The listing builds one solid part. Answer for the finished solid, in the listing's coordinates (mm). A direction names the side the tool comes from. Give positions to 0.01 mm unless a question says otherwise; leave off trailing zeros. Loops run counter-clockwise (first coordinate to the right, second up) from the corner with the lowest first, then second, coordinate; pieces in that order, holes last. Notation, with made-up numbers: M 25,69 L 84,69 A23 cw 84,79 Z; hole C 74,24 d3. An arc over 180 degrees is marked long. One line per item, written item: value. Start each with the question number.
Q1. A cutting plane is placed at A-A, the plane x = -1.25. Determine the outline of the cut face in (y, z), and give its area (3 significant figures).
Q2. For faces 5 (the cylindrical face through (2.84, -3.63, 0.22)), 6 (the cylindrical face through (-0.518, -0.045, 1.377)), 7 (the cylindrical face through (2.39, 0.07, -5.72)), 8 (the cylindrical face through (-1.644, -1.029, 1.643)), 9 (the flat face through (-6.422, 0, 1)), determine the directions among +Z, -Z, +X, -X, +Y, -Y from which every point of the face is accessible in a straight line to the end or side of a thin tool.
Q3. Flat-ended cylindrical pins translate along their axes: pin 1 (6 mm diameter, centred on x = 0, z = -0.956, fed in from -Y); pin 2 (1.6 mm diameter, centred on x = 4.5, y = 0, fed in from -Z); pin 3 (1.3 mm diameter, centred on x = 3.5, y = -1, fed in from +Z). Find the tip coordinate at first contact, or state that the pin passes through.
Q4. A cutting plane is placed at D-D, the plane x = 5.5. Determine the outline of the cut face in (y, z).
Q5. The mould has two halves that part along Z. Classify faces 1 (the flat face through (0, 0, -4.839)), 2 (the flat face through (0, 0, 4.839)), 3 (the flat face through (4, 0, -3.197)), 4 (the cylindrical face through (-1.567, 0.493, 3.219)): +Z half, -Z half, draft (parallel to the pull), parting line (faces both ways), or undercut.
Q6. A cutting plane is placed at C-C, the plane z = -3. Determine the outline of the cut face in (x, y) (1 decimal).
Q7. Consider L1, parallel to Y at x = -5, z = -2.25; L2, parallel to Z at x = 0, y = 3.8; L3, parallel to X at y = 0.25, z = 0.25 (1 decimal). Determine where each line is inside the solid, lowest interval first.
from build123d import *

# Parameters (mm, degrees)
SKETCH1_W                = 16.13
SKETCH1_H                = 9.678
BOSS_EXTRUDE1_DEPTH      = 8.065
SKETCH2_W                = 12.845
SKETCH2_H                = 4.78
CUT_EXTRUDE1_DEPTH       = 8.0355
BOSS_EXTRUDE2_DEPTH      = 4.78
SKETCH4_W                = 2.39
SKETCH4_H                = 1.78
SKETCH5_W                = 2.39
SKETCH5_H                = 1.78
SKETCH7_W                = 1.6425
SKETCH7_H                = 3.195419505
M3_CLEARANCE_HOLE1_D     = 3.285
M3_CLEARANCE_HOLE1_DEPTH = 1.78


with BuildPart() as part:
    # Sketch1 → Boss-Extrude1 (new body)
    with BuildSketch(Plane(origin=(0, 4.0325, 0), x_dir=(-1, 0, 0), z_dir=(0, 1, 0))):
        Rectangle(SKETCH1_W, SKETCH1_H)
    extrude(amount=-BOSS_EXTRUDE1_DEPTH)

    # Sketch2 → Cut-Extrude1 (cut)
    with BuildSketch(Plane.XY.offset(4.839)):
        Rectangle(SKETCH2_W, SKETCH2_H)
    extrude(amount=-CUT_EXTRUDE1_DEPTH, mode=Mode.SUBTRACT)

    # Sketch3 → Boss-Extrude2 (add)
    with BuildSketch(Plane.XZ.offset(-2.39)):
        with BuildLine():
            Line((2.106130278, -3.1965), (-2.106130278, -3.1965))
            ThreePointArc((-2.106130278, -3.1965), (0, 2.119), (2.106130278, -3.1965))
        make_face()
    extrude(amount=BOSS_EXTRUDE2_DEPTH)

    # Sketch4 → Revolve1 (revolve)
    with BuildSketch(Plane.XZ):
        with Locations((5.2275, -5.729)):
            Rectangle(SKETCH4_W, SKETCH4_H)
    revolve(axis=Axis((4.0325, 0, -4.839), (0, 0, -1)))

    # Sketch5 → Revolve2 (revolve)
    with BuildSketch(Plane.XZ):
        with Locations((-2.8375, -5.729)):
            Rectangle(SKETCH5_W, SKETCH5_H)
    revolve(axis=Axis((-4.0325, 0, -4.839), (0, 0, -1)))

    # Sketch6 → Cut-Revolve1 (revolve, cut)
    with BuildSketch(Plane(origin=(0, 0, -0.956), x_dir=(-1, 0, 0), z_dir=(0, 0, -1))):
        Polygon((-3.075, -4.0325), (0, -4.0325), (0, 4.0325), (-3.075, 4.0325), (-3.075, 3.2175), (-2.39, 3.2175), (-2.39, -3.2175), (-3.075, -3.2175), align=None)
    revolve(axis=Axis((0, -4.0325, -0.956), (0, 1, 0)), mode=Mode.SUBTRACT)

    # Sketch7 → Revolve3 (revolve)
    with BuildSketch(Plane(origin=(0, 0, 0), x_dir=(1, 0, 0), z_dir=(0, 1, 0))):
        with Locations((-0.82125, -3.241290248)):
            Rectangle(SKETCH7_W, SKETCH7_H)
    revolve(axis=Axis((0, 0, 4.839), (0, 0, -1)))

    # M3 Clearance Hole1
    with Locations(Plane(origin=(0, 0, -6.619), x_dir=(-1, 0, 0), z_dir=(0, 0, -1))):
        with Locations((4.0325, 0), (-4.0325, 0)):
            Hole(M3_CLEARANCE_HOLE1_D / 2, depth=M3_CLEARANCE_HOLE1_DEPTH)


solid = part.part
Answer block:
1. outline: M -4.03,-4.84 L 4.03,-4.84 L 4.03,-3.77 L 3.22,-3.77 L 3.22,-2.99 L -3.22,-2.99 L -3.22,-3.77 L -4.03,-3.77 Z; M -4.03,1.85 L -3.22,1.85 L -3.22,1.08 L 3.22,1.08 L 3.22,1.85 L 4.03,1.85 L 4.03,4.84 L 2.39,4.84 L 2.39,1.85 L 1.07,1.85 L 1.07,4.84 L -1.07,4.84 L -1.07,1.85 L -2.39,1.85 L -2.39,4.84 L -4.03,4.84 Z
1. area: 34.8 mm^2
2. face 5: -Y
2. face 6: +Y, -Y
2. face 7: -Z
2. face 8: none
2. face 9: +Z
3. pin 1: y = -3.22
3. pin 2: z = -4.84
3. pin 3: z = 0.2
4. outline: M -4.03,-4.84 L -1.89,-4.84 L -1.89,-6.62 L -0.74,-6.62 L -0.74,-4.84 L 0.74,-4.84 L 0.74,-6.62 L 1.89,-6.62 L 1.89,-4.84 L 4.03,-4.84 L 4.03,4.84 L 2.39,4.84 L 2.39,-3.2 L -2.39,-3.2 L -2.39,4.84 L -4.03,4.84 Z
5. face 1: -Z half
5. face 2: +Z half
5. face 3: undercut
5. face 4: draft
6. outline: M -8.1,-4 L -2.3,-4 L -2.3,-3.2 L -1.2,-3.2 L -1.2,3.2 L -2.3,3.2 L -2.3,4 L -8.1,4 Z; M 1.2,-3.2 L 2.3,-3.2 L 2.3,-4 L 8.1,-4 L 8.1,4 L 2.3,4 L 2.3,3.2 L 1.2,3.2 Z; hole M -6.4,-2.4 L -2.3,-2.4 L -2.3,2.4 L -6.4,2.4 Z; hole M 2.3,-2.4 L 6.4,-2.4 L 6.4,2.4 L 2.3,2.4 Z
7. L1: -4.03 to -2.39, 2.39 to 4.03
7. L2: -4.84 to -4.03, 2.12 to 4.84
7. L3: -8.1 to -6.4, -2.8 to -2.1, 2.1 to 2.8, 6.4 to 8.1
